Check sheet for the modelled part. Datum: model origin and axes. Units: mm. A direction names the side the tool comes from. Round coordinates to 2 decimals unless told otherwise and drop trailing zeros. Order: outer loops, then holes, each group sorted by start corner. A loop starts at its lowest first (then second) coordinate and runs counter-clockwise, first axis right, second up.
Q1. Cross-section at C-C on x = 0.5. Record the cut outline in (y, z).
Q2. Cross-section at A-A on z = 10.5. Record the cut outline in (x, y), then the cut area to 3 significant figures.
Q3. Cross-section at B-B on y = 14. Record the cut outline in (x, z), then the cut area to 3 significant figures.
Q4. Scan lines: probe 1 along X at (y, z) = (0, -1.05); probe 2 along Y at (x, z) = (0, 5.75); probe 3 along Z at (x, y) = (2.5, 19.5). Record each from-to range of solid material in increasing order.
Q5. Set-up check for faces 1 (the flat face through (5, 9, 7)), 2 (the cylindrical face through (4.007, 9.301, 20.715)), 3 (the cylindrical face through (1.049, 12.301, 12.715)): record each of +Z, -Z, +X, -X, +Y, -Y from which the full face is reachable in a straight line by a thin tool's end or side.
Q6. Depth check by flat-ended pin: P1, Ø3, axis at x = 10, z = 9, coming from the -Y side; P2, Ø12, axis at x = -23, z = 2, coming from the +Y side; P3, Ø3.5, axis at x = 0, y = 0, coming from the -Z side; P4, Ø2, axis at x = 7.5, y = 6.5, coming from the +Z side. Enter the tip coordinate at first touch or a pass-through.
Q7. Mould release check, pull along Z, two halves, no side actions. Record for faces 4 (the cylindrical face through (-2.785, 7.301, 6.874)), 5 (the flat face through (-10, -1, -2)), 6 (the flat face through (1, 17, 13)): +Z half, -Z half, draft (parallel to the pull), parting line (faces both ways), or undercut.
Q8. Cross-section at D-D on z = 13.5. Record the cut outline in (x, y).
from build123d import *
from build123d.topology import SkipClean

# Parameters (mm, degrees)
SKETCH_1_R          = 7
SKETCH_1_R_2        = 1.6
EXTRUDE_1_DEPTH     = 14
FILLET_2_R          = 1
FILLET_4_R          = 2
FILLET_5_R          = 1
CUT_EXTRUDE_1_DEPTH = 10
SKETCH_4_R          = 43
SKETCH_4_W          = 56
SKETCH_4_H          = 56
CUT_EXTRUDE_2_DEPTH = 2
SKETCH_5_R          = 1.6
EXTRUDE_3_DEPTH     = 2
EXTRUDE_START       = 2
SKETCH_6_R          = 1.6
EXTRUDE_4_DEPTH     = 2
EXTRUDE_START_2     = 1
EXTRUDE_6_DEPTH     = 1
EXTRUDE_7_DEPTH     = 1
EXTRUDE_8_DEPTH     = 8
CUT_EXTRUDE_3_DEPTH = 45.127655727
FILLET_6_R          = 1
EXTRUDE_10_DEPTH    = 1


with BuildPart() as part:
    # 草图1 → 凸台-拉伸1 (new body)
    # profile 1 of 3: a face of its own
    with BuildSketch(Plane.XY):
        with BuildLine():
            Line((-2.5, 7), (-20, 7))
            ThreePointArc((-20, 7), (-15.050252532, 4.949747468), (-13, 0))
            ThreePointArc((-13, 0), (-15.050252532, -4.949747468), (-20, -7))
            Line((-20, -7), (0, -7))
            ThreePointArc((0, -7), (-4.949747468, 4.949747468), (7, 0))
            Line((7, 0), (7, 4))
            Line((7, 4), (12, 4))
            Line((12, 4), (12, 5))
            Line((12, 5), (6.5, 9))
            Line((6.5, 9), (3.5, 9))
            Line((3.5, 9), (3.5, 26))
            Line((3.5, 26), (-2.5, 26))
            Line((-2.5, 26), (-2.5, 7))
        make_face()
    # profile 2 of 3: a face of its own
    with BuildSketch(Plane.XY):
        Circle(SKETCH_1_R)
        Circle(SKETCH_1_R_2, mode=Mode.SUBTRACT)
    # profile 3 of 3: a face of its own
    with BuildSketch(Plane.XY):
        with Locations((-20, 0)):
            Circle(SKETCH_1_R)
        with Locations((-20, 0)):
            Circle(SKETCH_1_R_2, mode=Mode.SUBTRACT)
    extrude(amount=EXTRUDE_1_DEPTH)

    # 圆角2
    fillet_2_edges = [part.edges().sort_by_distance(p)[0] for p in [
        (-2.5, 7, 7),
        (7, 4, 7),
    ]]
    fillet(fillet_2_edges, radius=FILLET_2_R)

    # 圆角4
    fillet_4_edges = [part.edges().sort_by_distance(p)[0] for p in [
        (6.5, 9, 7),
    ]]
    fillet(fillet_4_edges, radius=FILLET_4_R)

    # 圆角5
    fillet_5_edges = [part.edges().sort_by_distance(p)[0] for p in [
        (12, 5, 7),
    ]]
    fillet(fillet_5_edges, radius=FILLET_5_R)

    # 草图2 → 切除-拉伸1 (cut)
    with BuildSketch(Plane(origin=(3.5, 0, 0), x_dir=(0, 0, -1), z_dir=(1, 0, 0))):
        Polygon((-12, 9), (-14, 9), (-14, 26), (0, 26), (0, 9), (-2, 9), (-2, 24), (-12, 24), align=None)
    extrude(amount=-CUT_EXTRUDE_1_DEPTH, mode=Mode.SUBTRACT)

    # 草图4 → 切除-拉伸2 (cut)
    with BuildSketch(Plane.XY.offset(14)):
        with Locations((31.5, 37)):
            Circle(SKETCH_4_R)
        with Locations((31.5, 37)):
            Rectangle(SKETCH_4_W, SKETCH_4_H, mode=Mode.SUBTRACT)
    cut_extrude_2 = extrude(amount=-CUT_EXTRUDE_2_DEPTH, mode=Mode.SUBTRACT)

    # 镜向1: 切除-拉伸2 across plane
    add(cut_extrude_2.mirror(Plane.XY.offset(7)), mode=Mode.SUBTRACT)

    # 草图5 → 凸台-拉伸3 (add)
    with SkipClean():  # the faces are left unmerged after this step: merging them gives an invalid solid
        with BuildSketch(Plane.XY.offset(14)):
            with BuildLine():
                Line((-1.134337744, 9), (-2.5, 9))
                Line((-2.5, 9), (-2.5, 8))
                ThreePointArc((-2.5, 8), (-2.792893219, 7.292893219), (-3.5, 7))
                Line((-3.5, 7), (-20, 7))
                ThreePointArc((-20, 7), (-27, 0), (-20, -7))
                Line((-20, -7), (0, -7))
                ThreePointArc((0, -7), (4.949747468, -4.949747468), (7, 0))
                Line((7, 0), (7, 1.662343032))
                ThreePointArc((7, 1.662343032), (2.698204226, 5.071070168), (-1.134337744, 9))
            make_face()
            Circle(SKETCH_5_R, mode=Mode.SUBTRACT)
            with Locations((-20, 0)):
                Circle(SKETCH_5_R, mode=Mode.SUBTRACT)
        extrude(amount=EXTRUDE_3_DEPTH)

    # 草图6 → 凸台-拉伸4 (add)
    with SkipClean():  # the faces are left unmerged after this step: merging them gives an invalid solid
        with BuildSketch(Plane(origin=(0, 0, 0), x_dir=(-1, 0, 0), z_dir=(0, 0, -1)).offset(EXTRUDE_START)):
            with BuildLine():
                Line((-7, 1.662343032), (-7, 0))
                ThreePointArc((-7, 0), (-4.949747468, -4.949747468), (0, -7))
                Line((0, -7), (20, -7))
                ThreePointArc((20, -7), (27, 0), (20, 7))
                Line((20, 7), (3.5, 7))
                ThreePointArc((3.5, 7), (2.792893219, 7.292893219), (2.5, 8))
                Line((2.5, 8), (2.5, 9))
                Line((2.5, 9), (1.134337744, 9))
                ThreePointArc((1.134337744, 9), (-2.698204226, 5.071070168), (-7, 1.662343032))
            make_face()
            with Locations((20, 0)):
                Circle(SKETCH_6_R, mode=Mode.SUBTRACT)
            Circle(SKETCH_6_R, mode=Mode.SUBTRACT)
        extrude(amount=-EXTRUDE_4_DEPTH)

    # 草图8 → 凸台-拉伸6 (add)
    with SkipClean():  # the faces are left unmerged after this step: merging them gives an invalid solid
        with BuildSketch(Plane.XY.offset(12).offset(EXTRUDE_START_2)):
            with BuildLine():
                Line((-2.5, 9), (-1.134337744, 9))
                ThreePointArc((-1.134337744, 9), (2.698204226, 5.071070168), (7, 1.662343032))
                Line((7, 1.662343032), (7, 3))
                ThreePointArc((7, 3), (7.292893219, 3.707106781), (8, 4))
                Line((8, 4), (12, 4))
                Line((12, 4), (12, 4.490775408))
                ThreePointArc((12, 4.490775408), (11.891114947, 4.944553053), (11.588171698, 5.299511493))
                Line((11.588171698, 5.299511493), (7.025975768, 8.617472169))
                ThreePointArc((7.025975768, 8.617472169), (6.468120717, 8.901965344), (5.849632373, 9))
                Line((5.849632373, 9), (3.5, 9))
                Line((3.5, 9), (3.5, 24))
                Line((3.5, 24), (-2.5, 24))
                Line((-2.5, 24), (-2.5, 9))
            make_face()
        extrude(amount=-EXTRUDE_6_DEPTH)

    # 草图9 → 凸台-拉伸7 (add)
    with SkipClean():  # the faces are left unmerged after this step: merging them gives an invalid solid
        with BuildSketch(Plane(origin=(0, 0, 2), x_dir=(-1, 0, 0), z_dir=(0, 0, -1))):
            with BuildLine():
                Line((-3.5, 24), (-3.5, 9))
                Line((-3.5, 9), (-5.849632373, 9))
                ThreePointArc((-5.849632373, 9), (-6.468120717, 8.901965344), (-7.025975768, 8.617472169))
                Line((-7.025975768, 8.617472169), (-11.588171698, 5.299511493))
                ThreePointArc((-11.588171698, 5.299511493), (-11.891114947, 4.944553053), (-12, 4.490775408))
                Line((-12, 4.490775408), (-12, 4))
                Line((-12, 4), (-8, 4))
                ThreePointArc((-8, 4), (-7.292893219, 3.707106781), (-7, 3))
                Line((-7, 3), (-7, 1.662343032))
                ThreePointArc((-7, 1.662343032), (-2.698204226, 5.071070168), (1.134337744, 9))
                Line((1.134337744, 9), (2.5, 9))
                Line((2.5, 9), (2.5, 24))
                Line((2.5, 24), (-3.5, 24))
            make_face()
        extrude(amount=EXTRUDE_7_DEPTH)

    # 草图14 → 凸台-拉伸8 (add)
    with SkipClean():  # the faces are left unmerged after this step: merging them gives an invalid solid
        with BuildSketch(Plane.XY.offset(13)):
            Polygon((-1.134337744, 9), (3.5, 9), (3.5, 24), (-2.5, 24), (-2.5, 9), align=None)
        extrude(amount=EXTRUDE_8_DEPTH)

    # 草图13 → 切除-拉伸3 (cut, through all)
    with SkipClean():  # the faces are left unmerged after this step: merging them gives an invalid solid
        with BuildSketch(Plane(origin=(3.5, 0, 0), x_dir=(0, 0, -1), z_dir=(1, 0, 0))):
            with BuildLine():
                Line((-13, 20), (-13, 13))
                ThreePointArc((-13, 13), (-12.707106781, 12.292893219), (-12, 12))
                Line((-12, 12), (-5.5, 12))
                ThreePointArc((-5.5, 12), (-4.792893219, 12.292893219), (-4.5, 13))
                Line((-4.5, 13), (-4.5, 20))
                ThreePointArc((-4.5, 20), (-4.792893219, 20.707106781), (-5.5, 21))
                Line((-5.5, 21), (-12, 21))
                ThreePointArc((-12, 21), (-12.707106781, 20.707106781), (-13, 20))
            make_face()
        extrude(amount=-CUT_EXTRUDE_3_DEPTH, mode=Mode.SUBTRACT)

    # 圆角6
    fillet_6_edges = [part.edges().sort_by_distance(p)[0] for p in [
        (0.5, 24, 1),
        (0.5, 24, 21),
        (0.5, 9, 21),
    ]]
    fillet(fillet_6_edges, radius=FILLET_6_R - 0.0001)  # a hair under: the kernel refuses the full size

    # 草图16 → 凸台-拉伸10 (add)
    with SkipClean():  # the faces are left unmerged after this step: merging them gives an invalid solid
        with BuildSketch(Plane(origin=(3.5, 0, 0), x_dir=(0, 0, -1), z_dir=(1, 0, 0)).offset(EXTRUDE_START_2)):
            with BuildLine():
                Line((-1, 9), (-1, 23))
                ThreePointArc((-1, 23), (-1.292893219, 23.707106781), (-2, 24))
                Line((-2, 24), (-20, 24))
                ThreePointArc((-20, 24), (-20.707106781, 23.707106781), (-21, 23))
                Line((-21, 23), (-21, 10))
                ThreePointArc((-21, 10), (-20.707106781, 9.292893219), (-20, 9))
                Line((-20, 9), (-13, 9))
                Line((-13, 9), (-1, 9))
            make_face()
            with BuildLine():
                Line((-12, 12), (-5.5, 12))
                ThreePointArc((-5.5, 12), (-4.792893219, 12.292893219), (-4.5, 13))
                Line((-4.5, 13), (-4.5, 20))
                ThreePointArc((-4.5, 20), (-4.792893219, 20.707106781), (-5.5, 21))
                Line((-5.5, 21), (-12, 21))
                ThreePointArc((-12, 21), (-12.707106781, 20.707106781), (-13, 20))
                Line((-13, 20), (-13, 13))
                ThreePointArc((-13, 13), (-12.707106781, 12.292893219), (-12, 12))
            make_face(mode=Mode.SUBTRACT)
        extrude(amount=-EXTRUDE_10_DEPTH)


solid = part.part
Results found:
1. outline: (-6.98, -2) - (-1.52, -2) - (-1.52, 16) - (-6.98, 16) - close; (1.52, -2) - (7.2, -2) - (7.2, 1) - (23, 1) arc R1 ccw to (24, 2) - (24, 20) arc R1 ccw to (23, 21) - (10, 21) arc R1 ccw to (9, 20) - (9, 13) - (7.2, 13) - (7.2, 16) - (1.52, 16) - close; hole (12, 5.5) arc R1 ccw to (13, 4.5) - (20, 4.5) arc R1 ccw to (21, 5.5) - (21, 12) arc R1 ccw to (20, 13) - (13, 13) arc R1 ccw to (12, 12) - close
2. outline: (-20, -7) - (0, -7) arc R7 ccw to (7, 0) - (7, 3) arc R1 cw to (8, 4) - (12, 4) - (12, 4.49) arc R1 ccw to (11.59, 5.3) - (7.03, 8.62) arc R2 ccw to (5.85, 9) - (4.5, 9) - (4.5, 12) - (-2.5, 12) - (-2.5, 8) arc R1 cw to (-3.5, 7) - (-20, 7) arc R7 ccw to start; (-2.5, 21) - (4.5, 21) - (4.5, 24) - (-2.5, 24) - close; hole circle Ø3.2 at (-20, 0); hole circle Ø3.2 at (0, 0)
2. area: 504 mm2
3. outline: (-2.5, 1) - (4.5, 1) - (4.5, 4.5) - (-2.5, 4.5) - close; (-2.5, 13) - (4.5, 13) - (4.5, 21) - (-2.5, 21) - close
3. area: 80.5 mm2
4. probe 1: x = -27 to -21.6, -18.4 to -1.6, 1.6 to 7
4. probe 2: y = -7 to -1.6, 1.6 to 12, 21 to 24
4. probe 3: z = 1 to 4.5, 13 to 21
5. face 1: +Z, -Z, +X, +Y
5. face 2: +Z, +X, -X, -Y
5. face 3: +X, -X
6. P1: stops at y = 4
6. P2: stops at y = 7
6. P3: stops at z = -2
6. P4: stops at z = 13
7. face 4: draft
7. face 5: -Z half
7. face 6: undercut
8. outline: (-20, -7) - (0, -7) arc R7 ccw to (7, 0) - (7, 1.66) arc R43 cw to (-1.13, 9) - (4.5, 9) - (4.5, 24) - (-2.5, 24) - (-2.5, 8) arc R1 cw to (-3.5, 7) - (-20, 7) arc R7 ccw to start; hole circle Ø3.2 at (-20, 0); hole circle Ø3.2 at (0, 0)
